from build123d import *

# Parameters (mm, degrees)
SKETCH_1_W          = 32
SKETCH_1_H          = 27
EXTRUDE_1_DEPTH     = 18
SKETCH_2_R          = 12.5
CUT_EXTRUDE_1_DEPTH = 13.5
SKETCH_3_R          = 3.5
CUT_EXTRUDE_2_DEPTH = 4
SKETCH_4_R          = 0.95
CUT_EXTRUDE_3_DEPTH = 40.118409988
CUT_EXTRUDE_4_DEPTH = 28.608875443
CHAMFER_2_SIZE      = 1.5
CHAMFER_2_SIZE2     = 4.921659428
CHAMFER_4_SIZE      = 0.5


with BuildPart() as part:
    # 草图1 → 凸台-拉伸1 (new body)
    with BuildSketch(Plane(origin=(0, 0, 0), x_dir=(0, 0, -1), z_dir=(1, 0, 0))):
        Rectangle(SKETCH_1_W, SKETCH_1_H)
    extrude(amount=EXTRUDE_1_DEPTH)

    # 草图2 → 切除-拉伸1 (cut)
    with BuildSketch(Plane.ZY):
        Circle(SKETCH_2_R)
    extrude(amount=-CUT_EXTRUDE_1_DEPTH, mode=Mode.SUBTRACT)

    # 草图3 → 切除-拉伸2 (cut)
    with BuildSketch(Plane.ZY.offset(-13.5)):
        Circle(SKETCH_3_R)
    extrude(amount=-CUT_EXTRUDE_2_DEPTH, mode=Mode.SUBTRACT)

    # 草图4 → 切除-拉伸3 (cut, through all)
    with BuildSketch(Plane(origin=(0, 0, -16), x_dir=(-1, 0, 0), z_dir=(0, 0, -1))):
        with Locations((-14, 9.5)):
            Circle(SKETCH_4_R)
        with Locations((-4, 9.5)):
            Circle(SKETCH_4_R)
        with Locations((-4, -9.5)):
            Circle(SKETCH_4_R)
        with Locations(Location((-14, -9.5, 0), (0, 0, 180))):
            Circle(SKETCH_4_R)
    extrude(amount=-CUT_EXTRUDE_3_DEPTH, mode=Mode.SUBTRACT)

    # 草图6 → 切除-拉伸4 (cut, through all)
    with BuildSketch(Plane.ZY):
        with BuildLine():
            Line((16, -13.5), (16, 3.515112589))
            Line((16, 3.515112589), (12.507048233, -5.08170685))
            ThreePointArc((12.507048233, -5.08170685), (7.538134966, -11.199398253), (0, -13.5))
            Line((0, -13.5), (16, -13.5))
        make_face()
    extrude(amount=-CUT_EXTRUDE_4_DEPTH, mode=Mode.SUBTRACT)

    # 倒角2
    chamfer_2_edges = [part.edges().sort_by_distance(p)[0] for p in [
        (9, 3.515112589, 16),
    ]]
    chamfer_2_side = [part.faces().sort_by_distance(p)[0] for p in [
        (9, 8.475223706, 16),
    ]]
    chamfer(chamfer_2_edges, length=CHAMFER_2_SIZE, length2=CHAMFER_2_SIZE2, reference=chamfer_2_side[0])

    # 倒角3
    # the kernel refuses this chamfer: 1 mm, written as the material it takes off along each edge
    with BuildSketch(Plane(origin=(17.333333333, 12.833333333, 15.333333333), x_dir=(-0.7071067811865475, 0, 0.7071067811865475), z_dir=(0.5773502691896258, 0.5773502691896258, 0.5773502691896258)), Plane(origin=(17.333333333, 12.833333333, -15.333333333), x_dir=(-0.7071067811865475, 0.7071067811865475, 0), z_dir=(0.5773502691896258, 0.5773502691896258, -0.5773502691896258))) as chamfer_3_piece_1:
        Polygon((-0.707106781, 0.40824829), (0.707106781, 0.40824829), (0, -0.816496581), align=None)
    extrude(amount=1.270170592, mode=Mode.SUBTRACT)
    with BuildSketch(Plane(origin=(17.333333333, -12.833333333, -15.333333333), x_dir=(-0.7071067811865475, -0.7071067811865475, 0), z_dir=(0.5773502691896258, -0.5773502691896258, -0.5773502691896258))) as chamfer_3_piece_2:
        Polygon((-0.707106781, -0.40824829), (0.707106781, -0.40824829), (0, 0.816496581), align=None)
    extrude(amount=1.270170592, mode=Mode.SUBTRACT)
    with BuildSketch(Plane(origin=(18, 16.071682988, 16), x_dir=(-1, 0, 0), z_dir=(0, -1, 0)), Plane(origin=(0, 16.071682988, 16), x_dir=(0, 0, -1), z_dir=(0, -1, 0))) as chamfer_3_piece_3:
        with BuildLine():
            Line((1.028284271, -0.028284271), (-0.028284271, 1.028284271))
            Line((-0.028284271, 1.028284271), (-0.048284271, 1.028284271))
            ThreePointArc((-0.048284271, 1.028284271), (-0.02, 0.514142136), (-0.02, 0))
            Line((-0.02, 0), (0, -0.02))
            ThreePointArc((0, -0.02), (0.514142136, -0.02), (1.028284271, -0.048284271))
            Line((1.028284271, -0.048284271), (1.028284271, -0.028284271))
        make_face()
    extrude(amount=15.428431478, mode=Mode.SUBTRACT)
    with BuildSketch(Plane(origin=(18, -16.071682988, -16), x_dir=(-1, 0, 0), z_dir=(0, 1, 0)), Plane(origin=(0, -16.071682988, -16), x_dir=(0, 0, 1), z_dir=(0, 1, 0))) as chamfer_3_piece_4:
        with BuildLine():
            Line((1.028284271, -0.028284271), (-0.028284271, 1.028284271))
            Line((-0.028284271, 1.028284271), (-0.048284271, 1.028284271))
            ThreePointArc((-0.048284271, 1.028284271), (-0.02, 0.514142136), (-0.02, 0))
            Line((-0.02, 0), (0, -0.02))
            ThreePointArc((0, -0.02), (0.514142136, -0.02), (1.028284271, -0.048284271))
            Line((1.028284271, -0.048284271), (1.028284271, -0.028284271))
        make_face()
    extrude(amount=32.143365976, mode=Mode.SUBTRACT)
    with BuildSketch(Plane(origin=(18, -13.5, 0), x_dir=(-1, 0, 0), z_dir=(0, 0, -1))) as chamfer_3_piece_5:
        with BuildLine():
            Line((1.028284271, -0.028284271), (-0.028284271, 1.028284271))
            Line((-0.028284271, 1.028284271), (-0.048284271, 1.028284271))
            ThreePointArc((-0.048284271, 1.028284271), (-0.02, 0.514142136), (-0.02, 0))
            Line((-0.02, 0), (0, -0.02))
            ThreePointArc((0, -0.02), (0.514142136, -0.02), (1.028284271, -0.048284271))
            Line((1.028284271, -0.048284271), (1.028284271, -0.028284271))
        make_face()
    extrude(amount=18.571682988, mode=Mode.SUBTRACT)
    with BuildSketch(Plane(origin=(18, 0, 0), x_dir=(0, -1, 0), z_dir=(0, 0, -1))) as chamfer_3_piece_6:
        with BuildLine():
            Line((13.528284271, 1.028284271), (12.471715729, -0.028284271))
            Line((12.471715729, -0.028284271), (12.471715729, -0.048284271))
            ThreePointArc((12.471715729, -0.048284271), (12.985857864, -0.02), (13.5, -0.02))
            Line((13.5, -0.02), (13.52, 0))
            ThreePointArc((13.52, 0), (13.52, 0.514142136), (13.548284271, 1.028284271))
            Line((13.548284271, 1.028284271), (13.528284271, 1.028284271))
        make_face()
    revolve(axis=Axis((18, 0, 0), (-1, 0, 0)), revolution_arc=67.887726461, mode=Mode.SUBTRACT)
    with BuildSketch(Plane(origin=(18, -5.08170685, 12.507048233), x_dir=(-1, 0, 0), z_dir=(0, 0.9264480172326814, 0.3764227296081273))) as chamfer_3_piece_7:
        with BuildLine():
            Line((1.028284271, 0.028284271), (-0.028284271, -1.028284271))
            Line((-0.028284271, -1.028284271), (-0.048284271, -1.028284271))
            ThreePointArc((-0.048284271, -1.028284271), (-0.02, -0.514142136), (-0.02, 0))
            Line((-0.02, 0), (0, 0.02))
            ThreePointArc((0, 0.02), (0.514142136, 0.02), (1.028284271, 0.048284271))
            Line((1.028284271, 0.048284271), (1.028284271, 0.028284271))
        make_face()
    extrude(amount=17.216088275, mode=Mode.SUBTRACT)
    with BuildSketch(Plane(origin=(18, 9.195944132, 17.278208477), x_dir=(-1, 0, 0), z_dir=(0, -0.9563047559630353, -0.2923717047227372))) as chamfer_3_piece_8:
        with BuildLine():
            Line((1.028284271, -0.028284271), (-0.028284271, 1.028284271))
            Line((-0.028284271, 1.028284271), (-0.048284271, 1.028284271))
            ThreePointArc((-0.048284271, 1.028284271), (-0.02, 0.514142136), (-0.02, 0))
            Line((-0.02, 0), (0, -0.02))
            ThreePointArc((0, -0.02), (0.514142136, -0.02), (1.028284271, -0.048284271))
            Line((1.028284271, -0.048284271), (1.028284271, -0.028284271))
        make_face()
    extrude(amount=23.566814221, mode=Mode.SUBTRACT)
    with BuildSketch(Plane(origin=(-2.571682988, -13.5, -16), x_dir=(0, 0, 1), z_dir=(1, 0, 0))) as chamfer_3_piece_9:
        with BuildLine():
            Line((1.028284271, 0.028284271), (-0.028284271, -1.028284271))
            Line((-0.028284271, -1.028284271), (-0.048284271, -1.028284271))
            ThreePointArc((-0.048284271, -1.028284271), (-0.02, -0.514142136), (-0.02, 0))
            Line((-0.02, 0), (0, 0.02))
            ThreePointArc((0, 0.02), (0.514142136, 0.02), (1.028284271, 0.048284271))
            Line((1.028284271, 0.048284271), (1.028284271, 0.028284271))
        make_face()
    extrude(amount=23.143365976, mode=Mode.SUBTRACT)
    with BuildSketch(Plane(origin=(-2.571682988, 13.5, 16), x_dir=(0, -1, 0), z_dir=(1, 0, 0)), Plane(origin=(-2.571682988, 13.5, -16), x_dir=(0, 0, 1), z_dir=(1, 0, 0))) as chamfer_3_piece_10:
        with BuildLine():
            Line((1.028284271, -0.028284271), (-0.028284271, 1.028284271))
            Line((-0.028284271, 1.028284271), (-0.048284271, 1.028284271))
            ThreePointArc((-0.048284271, 1.028284271), (-0.02, 0.514142136), (-0.02, 0))
            Line((-0.02, 0), (0, -0.02))
            ThreePointArc((0, -0.02), (0.514142136, -0.02), (1.028284271, -0.048284271))
            Line((1.028284271, -0.048284271), (1.028284271, -0.028284271))
        make_face()
    extrude(amount=23.143365976, mode=Mode.SUBTRACT)
    with BuildSketch(Plane(origin=(18, 13.5, -18.571682988), x_dir=(-1, 0, 0), z_dir=(0, 0, 1))) as chamfer_3_piece_11:
        with BuildLine():
            Line((1.028284271, -0.028284271), (-0.028284271, 1.028284271))
            Line((-0.028284271, 1.028284271), (-0.048284271, 1.028284271))
            ThreePointArc((-0.048284271, 1.028284271), (-0.02, 0.514142136), (-0.02, 0))
            Line((-0.02, 0), (0, -0.02))
            ThreePointArc((0, -0.02), (0.514142136, -0.02), (1.028284271, -0.048284271))
            Line((1.028284271, -0.048284271), (1.028284271, -0.028284271))
        make_face()
    extrude(amount=37.143365976, mode=Mode.SUBTRACT)

    # 倒角4
    # the kernel refuses this chamfer: 0.5 mm, written as the material it takes off along each edge
    with BuildSketch(Plane(origin=(0, 13.5, -16.285841494), x_dir=(0, -1, 0), z_dir=(0, 0, 1))) as chamfer_4_piece_1:
        Polygon((CHAMFER_4_SIZE, 0), (0, CHAMFER_4_SIZE), (0, 0), align=None)
    extrude(amount=32.571682988, mode=Mode.SUBTRACT)
    with BuildSketch(Plane(origin=(0, 4.911777484, 16.567475349), x_dir=(0, 0.3764227296081273, -0.9264480172326813), z_dir=(0, -0.9264480172326814, -0.3764227296081273))) as chamfer_4_piece_2:
        Polygon((CHAMFER_4_SIZE, 0), (0, CHAMFER_4_SIZE), (0, 0), align=None)
    extrude(amount=10.786880805, mode=Mode.SUBTRACT)
    with BuildSketch(Plane(origin=(0, 0, 0), x_dir=(0, -0.3764227296081274, 0.9264480172326813), z_dir=(0, 0.9264480172326813, 0.3764227296081274))) as chamfer_4_piece_3:
        Polygon((13.5 - CHAMFER_4_SIZE, 0), (13.5, CHAMFER_4_SIZE), (13.5, 0), align=None)
    revolve(axis=Axis((0, 0, 0), (1, 0, 0)), revolution_arc=67.887726461, mode=Mode.SUBTRACT)
    with BuildSketch(Plane(origin=(0, -13.5, 0), x_dir=(0, 1, 0), z_dir=(0, 0, -1))) as chamfer_4_piece_4:
        Polygon((CHAMFER_4_SIZE, 0), (0, CHAMFER_4_SIZE), (0, 0), align=None)
    extrude(amount=16.285841494, mode=Mode.SUBTRACT)
    with BuildSketch(Plane(origin=(0, 0, 0), x_dir=(0, 0, 1), z_dir=(0, -1, 0))) as chamfer_4_piece_5:
        Polygon((12.5 + CHAMFER_4_SIZE, 0), (12.5, -CHAMFER_4_SIZE), (12.5, 0), align=None)
    revolve(axis=Axis((0, 0, 0), (-1, 0, 0)), mode=Mode.SUBTRACT)
    with BuildSketch(Plane(origin=(13.5, 0, 0), x_dir=(0, 0, 1), z_dir=(0, -1, 0))) as chamfer_4_piece_6:
        Polygon((3.5 + CHAMFER_4_SIZE, 0), (3.5, -CHAMFER_4_SIZE), (3.5, 0), align=None)
    revolve(axis=Axis((13.5, 0, 0), (-1, 0, 0)), mode=Mode.SUBTRACT)


solid = part.part
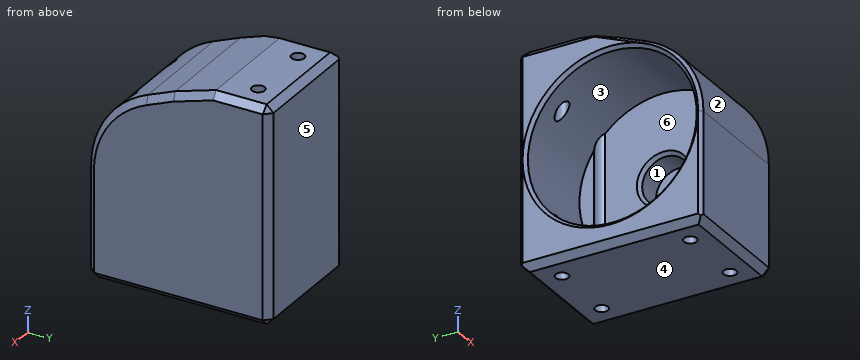
Geometry check sheet. Reference: the model listing, model coordinates, mm. Face numbers are marked on the shaded views. A direction names the side the tool comes from. Round coordinates to 2 decimals unless told otherwise and drop trailing zeros. Write each loop counter-clockwise with the first axis right and the second up, starting at its lowest first coordinate (ties: lowest second). Pieces come first, ordered by that corner, then holes.
Item 1: Mould release check, pull along Z, two halves, no side actions. Record for the marked faces 1, 2, 3 and 4: +Z half, -Z half, draft (parallel to the pull), parting line (faces both ways), or undercut.
Determined:
face 1: undercut
face 2: +Z half
face 3: undercut
face 4: -Z half
Item 2: Section check B-B (x = 4). Record the boundary of the cut face in (y, z).
Determined:
outline: (-13.5, -15) - (-12.5, -16) - (-10.45, -16) - (-10.45, -6.86) arc R12.5 cw to (-10.45, 6.86) - (-10.45, 8.55) arc R13.5 ccw to (-13.5, 0) - close; (-8.55, -16) - (8.55, -16) - (8.55, -9.12) arc R12.5 cw to (-8.55, -9.12) - close; (-8.55, 9.12) arc R12.5 cw to (8.55, 9.12) - (8.55, 16) - (5.02, 16) - (-1.04, 14.15) - (-5.08, 12.51) arc R13.5 ccw to (-8.55, 10.45) - close; (10.45, -16) - (12.5, -16) - (13.5, -15) - (13.5, 15) - (12.5, 16) - (10.45, 16) - (10.45, 6.86) arc R12.5 cw to (10.45, -6.86) - close
Item 3: Section check A-A (x = 15.5). Record the boundary of the cut face in (y, z), plus the area to 3 significant figures.
Determined:
outline: (-13.5, -15) - (-12.5, -16) - (12.5, -16) - (13.5, -15) - (13.5, 15) - (12.5, 16) - (5.02, 16) - (-1.04, 14.15) - (-5.08, 12.51) arc R13.5 ccw to (-13.5, 0) - close; hole circle Ø7 at (0, 0)
area: 749 mm2
Item 4: Go/stop test with flat-tipped pins: pin 1 Ø8.5 at (y, z) = (1.5, -5.5) entering from -X; pin 2 Ø2 at (x, y) = (4, -9.5) entering from +Z; pin 3 Ø3 at (x, y) = (4, 9.5) entering from +Z; pin 4 Ø3 at (x, z) = (8, 3.5) entering from -Y. Record where each tip stops, or that it passes through.
Determined:
pin 1: stops at x = 13.5
pin 2: stops at z = 10.49
pin 3: stops at z = 16
pin 4: stops at y = -13.35
Item 5: Section check C-C (y = 0). Record the boundary of the cut face in (x, z).
Determined:
outline: (0, -15) - (1, -16) - (17, -16) - (18, -15) - (18, 13.42) - (17, 14.47) - (0.4, 14.47) - (0, 14.03) - (0, 13) - (0.5, 12.5) - (13.5, 12.5) - (13.5, 4) - (14, 3.5) - (17.5, 3.5) - (17.5, -3.5) - (14, -3.5) - (13.5, -4) - (13.5, -12.5) - (0.5, -12.5) - (0, -13) - close
Item 6: Material ranges on line 1 along Y through (x, z) = (14, -6); line 2 along Y through (x, z) = (4, -10.5); line 3 along Y through (x, z) = (14, 7.5), recorded low to high.
Determined:
line 1: y = -13.5 to -10.45, -8.55 to 8.55, 10.45 to 13.5
line 2: y = -13.5 to -10.45, -8.55 to -6.78, 6.78 to 8.55, 10.45 to 13.5
line 3: y = -11.22 to -10.45, -8.55 to 8.55, 10.45 to 13.5
Item 7: Access from +Z, -Z, +X, -X, +Y, -Y to the whole of each face (thin tool, end or side, straight path). Record for the marked faces 5 and 6.
Determined:
face 5: +Z, -Z, +X, -X, +Y
face 6: -X
Item 8: Section check D-D (y = 9.5). Give the number of separate pieces and of enclosed holes in the cut face, plus the area to 3 significant figures.
Determined:
separate pieces: 5
enclosed holes: 0
area: 271 mm2
